Autodesk Inventor part; units mm, degrees
ref_plane "YZ Plane" through (0, 0, 0) normal (1, 0, 0) x (0, 1, 0)
ref_plane "XZ Plane" through (0, 0, 0) normal (0, 1, 0) x (-1, 0, 0)
ref_plane "XY Plane" through (0, 0, 0) normal (0, 0, 1) x (1, 0, 0)
sketch "Sketch1" plane through (0, 0, 0) normal (0, 1, 0) x (-1, 0, 0)
  circle A0 centre (0, 0) radius 5
  dimension "d0" = 10
extrude "Extrusion1" add sketch "Sketch1" along normal blind 100
sketch "Sketch2" plane through (0, 100, 0) normal (0, 1, 0) x (1, 0, 0)
  circle A0 centre (0, 0) radius 20
  dimension "d3" = 40
extrude "Extrusion2" add sketch "Sketch2" along normal blind 6
fillet "Fillet1" radius 2 1 edges at (5, 100, 0)
fillet "Fillet2" radius 5 1 edges at (5, 0, 0)
sketch "Sketch3" plane through (0, 106, 0) normal (0, 1, 0) x (1, 0, 0)
  point P0 (0, 0)
properties part number "Camera Holder"
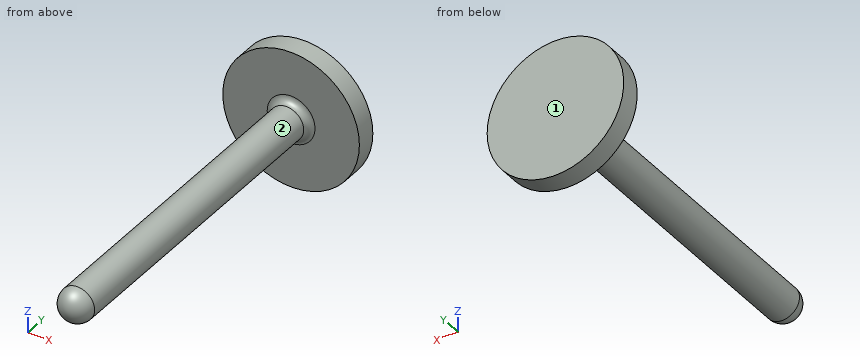
Work out the finished part from the listing and answer in its coordinate system (mm). Face numbers are marked on the shaded views. A direction names the side the tool comes from. Give positions to 0.01 mm unless a question says otherwise; leave off trailing zeros. Order: outer loops, then holes, each group sorted by start corner. A loop starts at its lowest first (then second) coordinate and runs counter-clockwise, first axis right, second up. Notation, with made-up numbers: (-12, 31) -> (14, 31) arc R27 ccw to (14, 63) -> close; hole circle Ø1 at (-15.75, 85). An arc over 180 degrees is marked (long way). Answer as CSV lines item,"result". Start each with the question number.
(1) Section D-D, the plane z = -12 is taken. Write down the section's boundary in (x, y), plus the area to 3 significant figures.
(2) Consider line 1 along Y through (x, z) = (-16.5, 1); line 2 along X through (y, z) = (102.5, 7) (3 decimals); line 3 along X through (y, z) = (62, 1). Determine where each line is inside the solid, lowest interval first.
(3) Each of these flat-tipped pins is pushed along its axis until it touches: pin 1 Ø4 at (x, z) = (7.5, 11.5) entering from -Y; pin 2 Ø8 at (x, y) = (2, 81.5) entering from -Z; pin 3 Ø6 at (y, z) = (44, 9.5) entering from +X; pin 4 Ø4 at (x, y) = (-4, 49) entering from -Z. Where does it stop, or does it pass through?
(4) Section A-A, the plane z = 0 is taken. Write down the section's boundary in (x, y), plus the area to 3 significant figures.
(5) Which of the six approach directions +Z, -Z, +X, -X, +Y, -Y give full straight-line access (tool end or side, diameter ignored) to the marked faces 1 and 2?
(6) Section C-C, the plane y = 42 is taken. Write down the section's boundary in (x, z).
(7) Section B-B, the plane x = 16 is taken. Write down the section's boundary in (y, z).
Entries:
1,outline,"(-16, 100) -> (16, 100) -> (16, 106) -> (-16, 106) -> close"
1,area,"192 mm²"
2,line 1,"100 to 106"
2,line 2,"-18.735 to 18.735"
2,line 3,"-4.9 to 4.9"
3,pin 1,"y = 100"
3,pin 2,"z = -5"
3,pin 3,"through"
3,pin 4,"z = -4.58"
4,outline,"(-20, 100) -> (-7, 100) arc R2 cw to (-5, 98) -> (-5, 5) arc R5 ccw to (5, 5) -> (5, 98) arc R2 cw to (7, 100) -> (20, 100) -> (20, 106) -> (-20, 106) -> close"
4,area,"1,230 mm²"
5,face 1,"+Z, -Z, +X, -X, +Y"
5,face 2,"-Y"
6,outline,"circle Ø10 at (0, 0)"
7,outline,"(100, -12) -> (106, -12) -> (106, 12) -> (100, 12) -> close"
